```python
from build123d import *

# Parameters (mm, degrees)
SKETCH1_W             = 25.4
SKETCH1_H             = 9.525
BOSS_EXTRUDE1_DEPTH   = 7.9375
BOSS_EXTRUDE2_DEPTH   = 15.875
CHAMFER1_SIZE         = 6.35
CHAMFER2_SIZE         = 3.175
CHAMFER2_SIZE2        = 2.93072295
F_8_CLEARANCE_HOLE1_D = 4.9149
CHAMFER3_SIZE         = 1.5875
BOSS_EXTRUDE3_DEPTH   = 3.429
BOSS_EXTRUDE4_START   = 3.175
SKETCH6_W             = 15.875
SKETCH6_H             = 20.446862299
SKETCH6_R             = 2.45745
BOSS_EXTRUDE4_DEPTH   = 3.175
SKETCH7_R             = 6.35
BOSS_EXTRUDE5_DEPTH   = 6.604
CUT_EXTRUDE1_DEPTH    = 44.214477453
CHAMFER5_SIZE         = 9.525


with BuildPart() as part:
    # Sketch1 → Boss-Extrude1 (new, symmetric)
    with BuildSketch(Plane(origin=(0, 0, 0), x_dir=(0, 0, -1), z_dir=(1, 0, 0))):
        Rectangle(SKETCH1_W, SKETCH1_H)
    extrude(amount=BOSS_EXTRUDE1_DEPTH, both=True)

    # Sketch2 → Boss-Extrude2 (add, through all)
    with BuildSketch(Plane.ZY.offset(7.9375)):
        Polygon((12.7, 4.7625), (37.438033761, 4.7625), (38.828997162, -11.13628443), (12.7, -11.13628443), align=None)
    extrude(amount=-BOSS_EXTRUDE2_DEPTH)

    # Chamfer1
    chamfer1_edges = [part.edges().sort_by_distance(p)[0] for p in [
        (7.9375, 0, -12.7),
        (7.9375, -7.949392215, 12.7),
        (-7.9375, -7.949392215, 12.7),
        (-7.9375, 0, -12.7),
    ]]
    chamfer(chamfer1_edges, length=CHAMFER1_SIZE)

    # Chamfer2
    chamfer2_edges = [part.edges().sort_by_distance(p)[0] for p in [
        (0, -11.13628443, 38.828997162),
    ]]
    chamfer2_side = [part.faces().sort_by_distance(p)[0] for p in [
        (0, -3.186892215, 38.133515462),
    ]]
    chamfer(chamfer2_edges, length=CHAMFER2_SIZE, length2=CHAMFER2_SIZE2, reference=chamfer2_side[0])

    # #8 Clearance Hole1 (through all)
    with Locations(Plane(origin=(0, -11.13628443, 0), x_dir=(-1, 0, 0), z_dir=(0, -1, 0))):
        with Locations((0, -25.62613884), (0, 0)):
            Hole(F_8_CLEARANCE_HOLE1_D / 2)

    # Chamfer3
    chamfer3_edges = [part.edges().sort_by_distance(p)[0] for p in [
        (0, -11.13628443, 12.7),
        (-7.9375, -11.13628443, 27.474137106),
        (7.9375, -11.13628443, 27.474137106),
        (-4.7625, -11.13628443, 15.875),
        (4.7625, -11.13628443, 15.875),
        (0, -4.7625, -12.7),
        (-4.7625, -4.7625, -9.525),
        (4.7625, -4.7625, -9.525),
        (-7.9375, -4.7625, 6.35),
        (7.9375, -4.7625, 6.35),
    ]]
    chamfer(chamfer3_edges, length=CHAMFER3_SIZE)

    # Sketch5 → Boss-Extrude3 (add)
    with BuildSketch(Plane(origin=(0, 4.7625, 0), x_dir=(1, 0, 0), z_dir=(0, 1, 0))):
        Polygon((4.5085, -37.438033761), (4.5085, -23.023155151), (0, -20.420171462), (-4.5085, -23.023155151), (-4.5085, -37.438033761), (-7.9375, -37.438033761), (-7.9375, -16.991171462), (7.9375, -16.991171462), (7.9375, -37.438033761), align=None)
    extrude(amount=BOSS_EXTRUDE3_DEPTH)

    # Sketch6 → Boss-Extrude4 (add)
    with BuildSketch(Plane(origin=(0, 8.1915, 0), x_dir=(1, 0, 0), z_dir=(0, 1, 0)).offset(BOSS_EXTRUDE4_START)):
        with Locations((0, -27.214602611)):
            Rectangle(SKETCH6_W, SKETCH6_H)
        with Locations(Location((0, -25.62613884, 0), (0, 0, 90))):
            Circle(SKETCH6_R, mode=Mode.SUBTRACT)
    extrude(amount=-BOSS_EXTRUDE4_DEPTH)

    # Sketch7 → Boss-Extrude5 (add)
    with BuildSketch(Plane(origin=(0, 4.7625, 0), x_dir=(1, 0, 0), z_dir=(0, 1, 0))):
        Polygon((-7.9375, 6.35), (-7.9375, -16.991171462), (7.9375, -16.991171462), (7.9375, 6.35), (1.5875, 12.7), (-1.5875, 12.7), align=None)
        with Locations(Location((0, 0, 0), (0, 0, 270))):
            Circle(SKETCH7_R, mode=Mode.SUBTRACT)
    extrude(amount=BOSS_EXTRUDE5_DEPTH)

    # Sketch8 → Cut-Extrude1 (cut, through all)
    with BuildSketch(Plane.ZY.offset(7.9375)):
        Polygon((37.438033761, 4.7625), (36.860258627, 11.3665), (37.438033761, 11.3665), align=None)
    extrude(amount=-CUT_EXTRUDE1_DEPTH, mode=Mode.SUBTRACT)

    # Chamfer5
    # the kernel refuses this chamfer: 9.525 mm, written as the material it takes off along each edge
    with BuildSketch(Plane(origin=(7.9375, -32.375434787, 40.687182042), x_dir=(0.027495876610586376, -0.08712279063518516, -0.9958180537233462), z_dir=(0, 0.9961946980917505, -0.0871557427476014))) as chamfer5_piece_1:
        Polygon((CHAMFER5_SIZE * 0.999621916911, CHAMFER5_SIZE * 0.0274958766106), (-CHAMFER5_SIZE * 0.0274958766106, CHAMFER5_SIZE * 0.999621916911), (0, 0), align=None)
    extrude(amount=68.404302332, mode=Mode.SUBTRACT)


solid = part.part
```
Work out the finished part from the listing and answer in its coordinate system (mm). A direction names the side the tool comes from. Give positions to 0.01 mm unless a question says otherwise; leave off trailing zeros. Order: outer loops, then holes, each group sorted by start corner. A loop starts at its lowest first (then second) coordinate and runs counter-clockwise, first axis right, second up. Notation, with made-up numbers: (4, 51.5) -> (44, 51.5) arc R27 cw to (44, 70.5) -> close; hole circle Ø8 at (24, -21). An arc over 180 degrees is marked (long way). Answer as CSV lines item,"result". Start each with the question number.
(1) Which of the six approach directions +Z, -Z, +X, -X, +Y, -Y give full straight-line access (tool end or side, diameter ignored) to faces 1 (the flat face through (0, 4.762, 29)), 2 (the flat face through (-7.13, -3.98, 6.17)), 3 (the flat face through (4.72, -7.11, 15.83)), 4 (the flat face through (0, -7, 12.7)), 5 (the flat face through (-4.72, 3.99, -9.57))?
(2) Section B-B, the plane y = -2.5 is taken. Write down the section's boundary in (x, z), plus the area to 3 significant figures.
(3) Consider line 1 along X through (y, z) = (4.25, 27.5); line 2 along X through (y, z) = (9.75, 0); line 3 along Z through (x, y) = (0, 1). Determine where each line is inside the solid, lowest interval first.
(4) Section D-D, the plane y = 7.25 is taken. Write down the section's boundary in (x, z), plus the area to 3 significant figures.
(5) For a pull along X with two mould halves and no side action, classify faces 6 (the cylindrical face through (-0.11, 9.8, 28.08)), 7 (the flat face through (7.13, -3.98, 6.53)), 8 (the flat face through (-7.155, -10.331, 28.267)) as released by +X, released by -X, zero draft, split by the parting line, or undercut.
(6) Each of these flat-tipped pins is pushed along its axis until it touches: pin 1 Ø1 at (x, z) = (4.5, 15.5) entering from -Y; pin 2 Ø4.5 at (x, z) = (0, 25.63) entering from +Y; pin 3 Ø7.5 at (x, z) = (0, 0) entering from +Y; pin 4 Ø8 at (x, y) = (4.5, 7.5) entering from +Z. Where does it stop, or does it pass through?
Entries:
1,face 1,"+Z"
1,face 2,"-Z, -X, -Y"
1,face 3,"-Z, +X, -Y"
1,face 4,"-Z, +X, -X, -Y"
1,face 5,"-Z, -X, +Y, -Y"
2,outline,"(-7.94, -6.35) -> (-1.59, -12.7) -> (1.59, -12.7) -> (7.94, -6.35) -> (7.94, 28.51) -> (-1.59, 38.07) -> (-7.94, 38.07) -> close; hole circle Ø4.91 at (0, 0); hole circle Ø4.91 at (0, 25.63)"
2,area,"682 mm²"
3,line 1,"-7.94 to -1.59, 1.59 to 7.94"
3,line 2,"-7.94 to -6.35, 6.35 to 7.94"
3,line 3,"-12.7 to -2.46, 2.46 to 23.17, 28.08 to 36.17"
4,outline,"(-7.94, -6.35) -> (-1.59, -12.7) -> (1.59, -12.7) -> (7.94, -6.35) -> (7.94, 27.66) -> (4.51, 31.1) -> (4.51, 23.02) -> (0, 20.42) -> (-4.51, 23.02) -> (-4.51, 37.22) -> (-7.94, 37.22) -> close; hole circle Ø12.7 at (0, 0)"
4,area,"459 mm²"
5,face 6,"undercut"
5,face 7,"released by +X"
5,face 8,"released by -X"
6,pin 1,"y = -9.97"
6,pin 2,"through"
6,pin 3,"y = 4.76"
6,pin 4,"z = 34.98"
